from build123d import *

# Parameters (mm, degrees)
SKETCH1_W           = 22
SKETCH1_H           = 22
SKETCH1_R           = 1.6
BOSS_EXTRUDE1_DEPTH = 10
SKETCH2_W           = 28
SKETCH2_H           = 20
BOSS_EXTRUDE2_DEPTH = 20
SKETCH3_W           = 7
SKETCH3_H           = 20
BOSS_EXTRUDE3_DEPTH = 20
SKETCH4_R           = 2.75
CUT_EXTRUDE1_DEPTH  = 12
SKETCH5_R           = 4.5
CUT_EXTRUDE2_DEPTH  = 11


with BuildPart() as part:
    # Sketch1 → Boss-Extrude1 (new body)
    with BuildSketch(Plane(origin=(0, 0, 0), x_dir=(1, 0, 0), z_dir=(0, 1, 0))):
        Rectangle(SKETCH1_W, SKETCH1_H)
        with Locations((-5.25, 5.25)):
            Circle(SKETCH1_R, mode=Mode.SUBTRACT)
        with Locations((6.25, 5.25)):
            Circle(SKETCH1_R, mode=Mode.SUBTRACT)
        with Locations((6.348618383, -6.25)):
            Circle(SKETCH1_R, mode=Mode.SUBTRACT)
        with Locations((-5.151381617, -6.25)):
            Circle(SKETCH1_R, mode=Mode.SUBTRACT)
    extrude(amount=BOSS_EXTRUDE1_DEPTH)

    # Sketch2 → Boss-Extrude2 (add)
    with BuildSketch(Plane(origin=(0, 0, -11), x_dir=(-1, 0, 0), z_dir=(0, 0, -1))):
        with Locations((3, 10)):
            Rectangle(SKETCH2_W, SKETCH2_H)
    extrude(amount=BOSS_EXTRUDE2_DEPTH)

    # Sketch3 → Boss-Extrude3 (add)
    with BuildSketch(Plane(origin=(0, 20, 0), x_dir=(1, 0, 0), z_dir=(0, 1, 0))):
        with Locations((-9.5, 21)):
            Rectangle(SKETCH3_W, SKETCH3_H)
    extrude(amount=BOSS_EXTRUDE3_DEPTH)

    # Sketch4 → Cut-Extrude1 (cut, through all)
    with BuildSketch(Plane(origin=(-6, 0, 0), x_dir=(0, 0, -1), z_dir=(1, 0, 0))):
        with Locations((21, 30)):
            Circle(SKETCH4_R)
    extrude(amount=-CUT_EXTRUDE1_DEPTH, mode=Mode.SUBTRACT)

    # Sketch5 → Cut-Extrude2 (cut, through all)
    with BuildSketch(Plane(origin=(0, 10, 0), x_dir=(1, 0, 0), z_dir=(0, 1, 0))):
        with Locations((0.5, -0.5)):
            Circle(SKETCH5_R)
    extrude(amount=-CUT_EXTRUDE2_DEPTH, mode=Mode.SUBTRACT)


solid = part.part
Input: part model. Units: mm. Frame: model coordinates. A direction names the side the tool comes from. Give positions to 0.01 mm unless a question says otherwise; leave off trailing zeros. Order: outer loops, then holes, each group sorted by start corner. A loop starts at its lowest first (then second) coordinate and runs counter-clockwise, first axis right, second up. Notation, with made-up numbers: M 56.25,81.25 L 68.25,81.25 A24 cw 68.25,102.25 Z; hole C 23.5,22 d8. An arc over 180 degrees is marked long. Answer as a JSON object with one key per item and string values.
1. Cut plane D-D, the plane x = -5.25. Output: boundary loops of the cut face in (y, z).
Result sheet:
{"outline": "M 0,-31 L 20,-31 L 20,-11 L 10,-11 L 10,-6.85 L 0,-6.85 Z; M 0,-3.65 L 10,-3.65 L 10,4.65 L 0,4.65 Z; M 0,7.85 L 10,7.85 L 10,11 L 0,11 Z"}
2. Pull-direction query (X, two-part tool) for faces 1 (the flat face through (-17, 10, -21)), 2 (the flat face through (-15, 20, -21)), 3 (the cylindrical face through (-6.52, 4.93, -4.28)); classes: +X half, -X half, draft (parallel to the pull), parting line (faces both ways), or undercut.
Result sheet:
{"face 1": "-X half", "face 2": "draft", "face 3": "undercut"}
3. First-contact query: P1, Ø16, axis at y = 31.5, z = -21.5, coming from the -X side; P2, Ø3, axis at x = 7.5, z = -18.5, coming from the +Y side; P3, Ø3, axis at y = 3, z = -0.5, coming from the -X side. Flat tips, straight axial feed; report the tip coordinate or a pass-through.
Result sheet:
{"P1": "x = -13", "P2": "y = 20", "P3": "x = -11"}
4. Cut plane B-B, the plane y = 30. Output: boundary loops of the cut face in (x, z).
Result sheet:
{"outline": "M -13,-31 L -6,-31 L -6,-23.75 L -13,-23.75 Z; M -13,-18.25 L -6,-18.25 L -6,-11 L -13,-11 Z"}
5. Ray query, line 1 (Z direction, x = -5.25, y = 5.5); line 2 (X direction, y = 6, z = -5.25); line 3 (X direction, y = 3, z = 6.25). Return the intervals inside material, ascending. Write a range as [from, to].
Result sheet:
{"line 1": "[-31, -6.85], [-3.65, 4.65], [7.85, 11]", "line 2": "[-11, -6.85], [-3.65, 4.65], [7.85, 11]", "line 3": "[-11, -6.75], [-3.55, 4.75], [7.95, 11]"}
6. Cut plane A-A, the plane z = 6.25. Output: boundary loops of the cut face in (x, y).
Result sheet:
{"outline": "M -11,0 L -6.75,0 L -6.75,10 L -11,10 Z; M -3.55,0 L 4.75,0 L 4.75,10 L -3.55,10 Z; M 7.95,0 L 11,0 L 11,10 L 7.95,10 Z"}
7. Reachability of faces 4 (the flat face through (-5, 10, 0)), 5 (the flat face through (-11, 5, 0)), 6 (the flat face through (3, 20, -21)), 7 (the flat face through (-6, 16, -11)), 8 (the flat face through (-13, 32.1, -18.6)) from +Z, -Z, +X, -X, +Y, -Y: full face, straight path, thin tool, end or side. Return the list, or none.
Result sheet:
{"face 4": "+Z, +X, -X, +Y", "face 5": "+Z, -X, +Y, -Y", "face 6": "+Z, -Z, +X, +Y", "face 7": "+Z, -X, +Y", "face 8": "+Z, -Z, -X, +Y"}
8. Cut plane C-C, the plane z = 0.5. Output: boundary loops of the cut face in (x, y).
Result sheet:
{"outline": "M -11,0 L -4,0 L -4,10 L -11,10 Z; M 5,0 L 11,0 L 11,10 L 5,10 Z"}
